Autodesk Inventor part; units mm, degrees
ref_plane "YZ Plane" through (0, 0, 0) normal (1, 0, 0) x (0, 1, 0)
ref_plane "XZ Plane" through (0, 0, 0) normal (0, 1, 0) x (-1, 0, 0)
ref_plane "XY Plane" through (0, 0, 0) normal (0, 0, 1) x (1, 0, 0)
sketch "Sketch1" plane through (0, 0, 0) normal (0, 1, 0) x (-1, 0, 0)
  line L0 (0, 0) -> (0, -48)
  line L1 (0, 0) -> (4.9, 0)
  line L2 (0, -24) -> (33, -24) construction
  line L3 (0, -48) -> (33, -48) construction
  line L4 (33, -48) -> (33, -43) construction
  line L5 (33, -48) -> (28, -48) construction
  line L6 (0, -48) -> (28, -48)
  line L7 (28, -48) -> (33, -43)
  line L8 (33, -43) -> (33, -23)
  line L9 (4.9, 0) -> (33, -23)
  dimension "d0" = 48
  dimension "d1" = 4.9
  dimension "d2" = 33
  dimension "d3" = 5
  dimension "d4" = 5
  dimension "d5" = 20
extrude "Extrusion1" add sketch "Sketch1" along normal blind 1
sketch "Sketch2" plane through (0, 1, 0) normal (0, 1, 0) x (1, 0, 0)
  line L0 (0, 0) -> (0, 48)
  line L1 (0, 48) -> (-28, 48)
  line L2 (-28, 48) -> (-33, 43)
  line L3 (-33, 43) -> (-33, 23)
  line L4 (-33, 23) -> (-4.9, 0)
  line L5 (-4.9, 0) -> (0, 0)
  line L6 (-5.9712, -3) -> (-36, 21.5787)
  line L7 (-36, 21.5787) -> (-36, 44.2426)
  line L8 (-36, 44.2426) -> (-29.2426, 51)
  line L9 (-29.2426, 51) -> (3, 51)
  line L10 (3, 51) -> (3, -3)
  line L11 (3, -3) -> (-5.9712, -3)
  dimension "d8" = 3
extrude "Extrusion2" add sketch "Sketch2" along normal blind 3 contours L5 L4 L3 L2 L1 L0 | L6 L7 L8 L9 L10 L11
sketch "Sketch3" plane through (0, 0, 0) normal (0, -1, 0) x (1, 0, 0)
  line L0 (0, 0) -> (0, -48)
  line L1 (-4.9, 0) -> (0, 0)
  line L2 (-33, -23) -> (-4.9, 0)
  line L3 (-33, -43) -> (-33, -23)
  line L4 (-28, -48) -> (-33, -43)
  line L5 (0, -48) -> (-28, -48)
  line L6 (3, -51) -> (3, 3)
  line L7 (3, 3) -> (-5.9712, 3)
  line L8 (-5.9712, 3) -> (-36, -21.5787)
  line L9 (-36, -21.5787) -> (-36, -44.2426)
  line L10 (-36, -44.2426) -> (-29.2426, -51)
  line L11 (-29.2426, -51) -> (3, -51)
  dimension "d11" = 3
extrude "Extrusion3" add sketch "Sketch3" along normal blind 3 contours L0 L5 L4 L3 L2 L1 | L11 L10 L9 L8 L7 L6
sketch "Sketch4" plane through (0, 0, 0) normal (0, 1, 0) x (1, 0, 0)
  line L0 (3, 51) -> (3, -3)
  line L1 (-29.2426, 51) -> (3, 51)
  line L2 (-36, 44.2426) -> (-29.2426, 51)
  line L3 (-36, 21.5787) -> (-36, 44.2426)
  line L4 (-5.9712, -3) -> (-36, 21.5787)
  line L5 (3, -3) -> (-5.9712, -3)
  line L6 (-4.9, 0) -> (0, 0)
  line L7 (-33, 23) -> (-4.9, 0)
  line L8 (-33, 43) -> (-33, 23)
  line L9 (-28, 48) -> (-33, 43)
  line L10 (0, 48) -> (-28, 48)
  line L11 (0, 0) -> (0, 48)
  line L12 (0, 0) -> (0, 48)
  line L13 (0, 48) -> (0, 51)
  line L14 (0, 0) -> (0, -3)
  line L15 (3, -3) -> (-5.9712, -3)
extrude "Extrusion4" add sketch "Sketch4" along normal blind 8 contours L13 L10 L9 L8 L7 L6 L14 L5 L4 L3 L2 L1
sketch "Sketch5" plane through (-36, 4, -44.2426) normal (-1, 0, 0) x (0, 0, 1)
  line L0 (0, 4) -> (0, -7)
  line L1 (22.6639, -7) -> (0, -7)
  line L2 (22.6639, 4) -> (22.6639, -7)
  line L3 (0, 4) -> (22.6639, 4)
  point P0 (44.2426, -4)
extrude "Extrusion5" add sketch "Sketch5" along normal blind 130
fillet "Fillet1" radius 2 6 edges at (-36, 2.5, -44.2426) (-36, 2.5, -21.5787) (-5.9712, 2.5, 3) (-29.2426, 2.5, -51) (-166, 2.5, -44.2426) (-166, 2.5, -21.5787)
sketch "Sketch6" plane through (0, 0, 0) normal (0, 1, 0) x (1, 0, 0)
  line L0 (0, -3) -> (0, 51)
  line L1 (3, -3) -> (0, -3)
  line L2 (3, 51) -> (3, -3)
  line L3 (0, 51) -> (3, 51)
  point P0 (0, 0)
extrude "Extrusion6" cut sketch "Sketch6" along normal blind 130 and the other way blind 65
sketch "Sketch7" plane through (0, 4, 0) normal (0, 1, 0) x (1, 0, 0)
  line L0 (0, 0) -> (0, 48)
  line L1 (0, 48) -> (-28, 48)
  line L2 (-28, 48) -> (-33, 43)
  line L3 (-33, 43) -> (-33, 23)
  line L4 (-33, 23) -> (-4.9, 0)
  line L5 (-4.9, 0) -> (0, 0)
extrude "Extrusion7" cut sketch "Sketch7" against normal blind 4
sketch "Sketch8" plane through (0, -3, 3) normal (1, 0, 0) x (0, 0, -1)
  point P0 (3, 3)
sketch "Sketch9" plane through (0, 8, 0) normal (0, 1, 0) x (1, 0, 0)
  line L0 (0, 48) -> (0, 0)
  line L1 (-28, 48) -> (0, 48)
  line L2 (-33, 43) -> (-28, 48)
  line L3 (-33, 23) -> (-33, 43)
  line L4 (-4.9, 0) -> (-33, 23)
  line L5 (0, 0) -> (-4.9, 0)
  arc A0 (-166, 23.5787) -> (-164, 21.5787) centre (-164, 23.5787) ccw
  line L6 (-36.7141, 21.5787) -> (-164, 21.5787)
  arc A1 (-35.4474, 21.1264) -> (-36.7141, 21.5787) centre (-36.7141, 19.5787) ccw
  line L7 (-35.4474, 21.1264) -> (-6.5238, -2.5477)
  arc A2 (-6.5238, -2.5477) -> (-5.2571, -3) centre (-5.2571, -1) ccw
  line L8 (-5.2571, -3) -> (0, -3)
  line L9 (0, -3) -> (0, 0)
  line L10 (0, 0) -> (-4.9, 0)
  line L11 (-4.9, 0) -> (-33, 23)
  line L12 (-33, 23) -> (-33, 43)
  line L13 (-33, 43) -> (-28, 48)
  line L14 (-28, 48) -> (0, 48)
  line L15 (0, 48) -> (0, 51)
  line L16 (0, 51) -> (-28.4142, 51)
  arc A3 (-28.4142, 51) -> (-29.8284, 50.4142) centre (-28.4142, 49) ccw
  line L17 (-29.8284, 50.4142) -> (-35.4142, 44.8284)
  arc A4 (-36.8284, 44.2426) -> (-35.4142, 44.8284) centre (-36.8284, 46.2426) ccw
  line L18 (-36.8284, 44.2426) -> (-164, 44.2426)
  arc A5 (-164, 44.2426) -> (-166, 42.2426) centre (-164, 42.2426) ccw
  line L19 (-166, 23.5787) -> (-166, 42.2426)
extrude "Extrusion8" add sketch "Sketch9" along normal blind 3
properties part number "PATAS"
Design review of the part built by this model. Coordinates are the model's own, in mm. A direction names the side the tool comes from. Coordinates: 2 decimals unless noted, no trailing zeros. Order: outer loops, then holes, each group sorted by start corner. A loop starts at its lowest first (then second) coordinate and runs counter-clockwise, first axis right, second up. Notation, with made-up numbers: (2, -40) -> (46, -40) arc R25 cw to (46, -7) -> close; hole circle Ø3 at (-24, -16). An arc over 180 degrees is marked (long way). One line per item, written item: value. Start each with the question number.
Q1. Mouldability with a two-part tool opening along Z and no side actions: class faces 4 (the flat face through (-30, 4, -46)), 5 (the flat face through (-99, 4, -21.579)), 6 (the flat face through (0, -1, -24)) as pulls with the +Z half, pulls with the -Z half, needs draft (parallel to the pull), parting line crosses it, or undercut.
Q2. Take a section at B-B, the plane x = -81.5. State the section outline as (y, z) points.
Q3. For probe 1 along Y at (x, z) = (-12, -23.5); probe 2 along Z at (x, y) = (-114, 0.75); probe 3 along Z at (x, y) = (-28, 6.5), list the stretches that pass through material, from the lowest coordinate up.
Q4. Take a section at C-C, the plane z = -7. State the section outline as (x, y) points.
Q5. Insertion check: pin 1 Ø3 at (y, z) = (4.5, -42.5) entering from +X; pin 2 Ø5 at (x, y) = (-34.5, 9.5) entering from -Z; pin 3 Ø7 at (x, y) = (-79, 6) entering from -Z. Each pin has a flat end and moves straight along its axis. Give the tip position at first contact, or say it passes through.
Q6. Tool access review of faces 1 (the flat face through (-100, 4, -44.243)), 2 (the flat face through (-66, 11, -30)), 3 (the flat face through (-13, 8, -30)): name each direction out of +Z, -Z, +X, -X, +Y, -Y from which nothing blocks a thin tool from reaching the whole face with its end or side.
Q7. Take a section at D-D, the plane z = -16.5. State the section outline as (x, y) points.
Q8. Take a section at A-A, the plane z = -40. State the section outline as (x, y) points.
Values follow:
1. face 4: undercut
1. face 5: pulls with the +Z half
1. face 6: needs draft
2. outline: (-3, -44.24) -> (11, -44.24) -> (11, -21.58) -> (-3, -21.58) -> close
3. probe 1: y = -3 to 0, 8 to 11
3. probe 2: z = -44.24 to -21.58
3. probe 3: z = -51 to -48, -18.91 to -15.03
4. outline: (-18.19, -3) -> (0, -3) -> (0, 0) -> (-13.45, 0) -> (-13.45, 8) -> (0, 8) -> (0, 11) -> (-18.19, 11) -> close
5. pin 1: stops at x = -32
5. pin 2: stops at z = -48.24
5. pin 3: stops at z = -44.24
6. face 1: -Z, -X, +Y, -Y
6. face 2: +Z, -Z, +X, -X, +Y
6. face 3: +X
7. outline: (-29.8, -3) -> (0, -3) -> (0, 0) -> (-25.06, 0) -> (-25.06, 8) -> (0, 8) -> (0, 11) -> (-29.8, 11) -> close
8. outline: (-166, -3) -> (0, -3) -> (0, 0) -> (-33, 0) -> (-33, 8) -> (0, 8) -> (0, 11) -> (-166, 11) -> close
